Autodesk Inventor part; units mm, degrees
ref_plane "YZ Plane" through (0, 0, 0) normal (1, 0, 0) x (0, 1, 0)
ref_plane "XZ Plane" through (0, 0, 0) normal (0, 1, 0) x (-1, 0, 0)
ref_plane "XY Plane" through (0, 0, 0) normal (0, 0, 1) x (1, 0, 0)
sketch "Sketch1" plane through (0, 0, 0) normal (0, 0, 1) x (1, 0, 0)
  line L0 (0, 0) -> (50, 0)
  line L1 (50, 0) -> (50, 52.5)
  line L2 (50, 52.5) -> (0, 52.5)
  line L3 (0, 52.5) -> (0, 0)
  dimension "d0" = 50
  dimension "d1" = 52.5
extrude "Extrusion1" add sketch "Sketch1" along normal blind 3
sketch "Sketch2" plane through (0, 0, 3) normal (0, 0, 1) x (1, 0, 0)
  line L0 (2, 50.5) -> (48, 50.5)
  line L1 (48, 50.5) -> (48, 2)
  line L2 (48, 2) -> (2, 2)
  line L3 (2, 2) -> (2, 50.5)
  dimension "d4" = 46
  dimension "d5" = 48.5
extrude "Extrusion2" cut sketch "Sketch2" against normal blind 10
sketch "Sketch5" plane through (0, 0, 0) normal (0, -1, 0) x (1, 0, 0)
  line L0 (12.85, 2.5) -> (12.85, 1.5)
  line L1 (2.85, 1.5) -> (2.85, 2.5)
  line L2 (0, 0) -> (50, 0)
  line L3 (14.1, 2.5) -> (14.966, 2)
  line L4 (14.966, 2) -> (14.1, 1.5)
  line L5 (14.1, 1.5) -> (14.1, 2.5)
  line L6 (2, 3) -> (48, 3)
  line L7 (1.35, 2.5) -> (0.35, 2.5)
  line L8 (0.35, 2.5) -> (0.35, 1.5)
  line L9 (0.35, 1.5) -> (1.35, 1.5)
  line L10 (1.35, 1.5) -> (1.35, 2.5)
  dimension "d24" = 1
  dimension "d25" = 1
  dimension "d26" = 1.5
  dimension "d27" = 1.25
  dimension "d28" = 1
  dimension "d29" = 1
  dimension "d30" = 1
  dimension "d31" = 1
  dimension "d32" = 1
  dimension "d33" = 0.5
  dimension "d34" = 1.5
extrude "Extrusion5" add sketch "Sketch5" along normal blind 4
chamfer "Chamfer3" distance 0.288 angle 45 3 edges at (14.533, -4, 1.75) (14.1, -4, 2) (14.533, -4, 2.25)
chamfer "Chamfer4" distance 0.288 angle 45 3 edges at (14.533, -3.712, 1.75) (14.1, -3.712, 2) (14.533, -3.712, 2.25)
chamfer "Chamfer5" distance 0.499 angle 45 4 edges at (0.85, -4, 1.5) (1.35, -4, 2) (0.85, -4, 2.5) (0.35, -4, 2)
chamfer "Chamfer6" distance 0.499 angle 45 4 edges at (0.85, -3.501, 1.5) (1.35, -3.501, 2) (0.85, -3.501, 2.5) (0.35, -3.501, 2)
sketch "Sketch8" plane through (0, 52.5, 0) normal (0, 1, 0) x (1, 0, 0)
  line L0 (50, 0) -> (0, 0)
  line L1 (50, 0) -> (50, -3)
  line L2 (13.7626, -1) -> (14.6286, -1.5)
  line L3 (13.7626, -1) -> (14.7626, -1) construction
  line L4 (14.6286, -1.5) -> (13.7626, -2)
  line L5 (12.66, -2.77) -> (12.66, -0.23)
  line L6 (13.7626, -2) -> (13.7626, -1)
  line L7 (13.5765, -2.1075) -> (13.5765, -0.8925)
  line L8 (13.5765, -0.8925) -> (13.5765, -0.7425)
  line L9 (13.5765, -0.7425) -> (14.8884, -1.5)
  line L10 (13.5765, -2.1075) -> (13.5765, -2.2575)
  line L11 (13.5765, -2.2575) -> (14.8884, -1.5)
  dimension "d60" = 1
  dimension "d61" = 30
  dimension "d62" = 1
  dimension "d63" = 60
  dimension "d64" = 1
  dimension "d65" = 35.3714
  dimension "d66" = 0.15
  dimension "d67" = 60
  dimension "d68" = 0.15
extrude "Extrusion8" add sketch "Sketch8" along normal blind 4
chamfer "Chamfer7" distance 0.12 angle 45 3 edges at (14.1956, 56.5, 1.75) (13.7626, 56.5, 1.5) (14.1956, 56.5, 1.25)
sketch "Sketch9" plane through (0, 52.5, 0) normal (0, 1, 0) x (1, 0, 0)
  line L0 (50, 0) -> (0, 0)
  line L1 (0, 0) -> (0, -3)
  line L2 (50, -3) -> (0, -3)
  line L3 (2, -2.77) -> (2, -0.23)
  line L4 (1.5, -2) -> (0.5, -2)
  line L5 (0.5, -2) -> (0.5, -1)
  line L6 (0.5, -1) -> (1.5, -1)
  line L7 (1.5, -1) -> (1.5, -2)
  line L8 (1.6, -2.1) -> (0.4, -2.1)
  line L9 (0.4, -2.1) -> (0.4, -0.9)
  line L10 (0.4, -0.9) -> (1.6, -0.9)
  line L11 (1.6, -0.9) -> (1.6, -2.1)
  dimension "d74" = 1
  dimension "d75" = 1
  dimension "d76" = 0.5
  dimension "d77" = 1
  dimension "d78" = 1
  dimension "d79" = 0.5
  dimension "d81" = 1.2
  dimension "d82" = 1.2
extrude "Extrusion9" add sketch "Sketch9" along normal blind 4
chamfer "Chamfer8" distance 0.1 angle 45 4 edges at (1.5, 56.5, 1.5) (1, 56.5, 2) (0.5, 56.5, 1.5) (1, 56.5, 1)
chamfer "Chamfer9" distance 0.1 angle 45 4 edges at (0.5, 56.4005, 1.5) (1, 56.4005, 2) (1.5, 56.4005, 1.5) (1, 56.4005, 1)
chamfer "Chamfer10" distance 0.1 angle 45 3 edges at (14.1956, 56.38, 1.75) (13.7626, 56.38, 1.5) (14.1956, 56.38, 1.25)
properties part number "Zijplaat 1.1"
Can you work these out from the model? Positions are in its coordinate system, mm. A direction names the side the tool comes from. Coordinates: 2 decimals unless noted, no trailing zeros. Loops run counter-clockwise (first coordinate to the right, second up) from the corner with the lowest first, then second, coordinate; pieces in that order, holes last.
Item 1: Suppose I cut it at B-B (x = 32). Please give me the cut outline in (y, z).
Answers below:
outline: (0, 0) - (2, 0) - (2, 3) - (0, 3) - close; (50.5, 0) - (52.5, 0) - (52.5, 3) - (50.5, 3) - close
Item 2: If we mould it in two halves opening along X, with no side actions, what happens to faces 1 (the face through (48, 27, 2)), 2 (the face through (1, 26, 3)), 3 (the face through (50, 26, 1))? For each: released by +X, released by -X, zero draft, split by the parting line, or undercut.
Answers below:
face 1: undercut
face 2: zero draft
face 3: released by +X
Item 3: I'm going to push flat-ended pins straight in: pin 1 (1.1 mm diameter, centred on y = 54.5, z = 1.5, fed in from +X); pin 2 (1 mm diameter, centred on x = 1, y = 55, fed in from +Z); pin 3 (1.1 mm diameter, centred on x = 1, y = -1, fed in from +Z). Where does each tip first touch, or does it pass through?
Answers below:
pin 1: stops at x = 14.89
pin 2: stops at z = 2.1
pin 3: stops at z = 2.5
Item 4: Please list where these lines run through material, in increasing order: L1, parallel to Y at x = 45.5, z = 1.55; L2, parallel to X at y = 38.5, z = 0.6.
Answers below:
L1: y = 0 to 2, 50.5 to 52.5
L2: x = 0 to 2, 48 to 50
Item 5: Suppose I cut it at A-A (y = 26). Please give me the cut outline in (x, z).
Answers below:
outline: (0, 0) - (2, 0) - (2, 3) - (0, 3) - close; (48, 0) - (50, 0) - (50, 3) - (48, 3) - close
Item 6: Which directions (+Z, -Z, +X, -X, +Y, -Y) give clear straight access to the entire face, cutting with the end or side of a thin tool? Please do faces 4 (the face through (13.576, 54, 2)), 5 (the face through (2, 26, 2)), 6 (the face through (1, 26, 0)).
Answers below:
face 4: +Z, -Z, +Y
face 5: +Z, -Z
face 6: -Z, +X, -X, +Y, -Y
